Work out the finished part from the listing and answer in its coordinate system (mm). Coordinates: 2 decimals unless noted, no trailing zeros. Order: outer loops, then holes, each group sorted by start corner. A loop starts at its lowest first (then second) coordinate and runs counter-clockwise, first axis right, second up. Notation, with made-up numbers: M 79.5,9 L 102.5,9 A18 ccw 102.5,28 Z; hole C 41,-11 d3. An arc over 180 degrees is marked long. Use a Markdown table: item, result.
from build123d import *

# Parameters (mm, degrees)
SKETCH001_R     = 26
PAD_DEPTH       = 20
SKETCH002_R     = 15
POCKET_DEPTH    = 20.001
SKETCH_R        = 4
POCKET001_DEPTH = 26


with BuildPart() as part:
    # Sketch001 → Pad (new body)
    with BuildSketch(Plane.XY):
        Circle(SKETCH001_R)
    extrude(amount=PAD_DEPTH)

    # Sketch002 (on Face3 of Pad) → Pocket (cut, through all)
    with BuildSketch(Plane.XY.offset(20)):
        Circle(SKETCH002_R)
    extrude(amount=-POCKET_DEPTH, mode=Mode.SUBTRACT)

    # Sketch (on DatumPlane) → Pocket001 (cut)
    with BuildSketch(Plane.XZ.offset(26)):
        with Locations((0, 10)):
            Circle(SKETCH_R)
    extrude(amount=-POCKET001_DEPTH, mode=Mode.SUBTRACT)


solid = part.part
(1) A cutting plane is placed at B-B (x = 0). Determine the outline of the cut face in (y, z), then the cut area to 3 significant figures.
Conclusion:
| item | result |
|---|---|
| outline | M -26,0 L -15,0 L -15,6 L -26,6 Z; M -26,14 L -15,14 L -15,20 L -26,20 Z; M 15,0 L 26,0 L 26,20 L 15,20 Z |
| area | 352 mm2 |
(2) Given P1, Ø2, axis at y = -7, z = 9.5, coming from the +X side; P2, Ø10, axis at x = -15, z = 10, coming from the -Y side; P3, Ø10, axis at x = -9, z = 8.5, coming from the -Y side, each flat-ended and moving along its own axis, determine where each tip first touches the part or whether it passes through.
Conclusion:
| item | result |
|---|---|
| P1 | x = 25.3 |
| P2 | y = -24 |
| P3 | y = -25.69 |
(3) A cutting plane is placed at A-A (y = 0). Determine the outline of the cut face in (x, z).
Conclusion:
| item | result |
|---|---|
| outline | M -26,0 L -15,0 L -15,20 L -26,20 Z; M 15,0 L 26,0 L 26,20 L 15,20 Z |
(4) Straight lines are drawn through the part: L1, parallel to Y at x = -0.5, z = 1.75; L2, parallel to Z at x = 0, y = -18; L3, parallel to X at y = 12, z = 13.5. For each, find the intervals that lie inside material, in ascending order.
Conclusion:
| item | result |
|---|---|
| L1 | -26 to -14.99, 14.99 to 26 |
| L2 | 0 to 6, 14 to 20 |
| L3 | -23.07 to -9, 9 to 23.07 |
(5) A cutting plane is placed at C-C (x = -10.5). Determine the outline of the cut face in (y, z), then the cut area to 3 significant figures.
Conclusion:
| item | result |
|---|---|
| outline | M -23.79,0 L -10.71,0 L -10.71,20 L -23.79,20 Z; M 10.71,0 L 23.79,0 L 23.79,20 L 10.71,20 Z |
| area | 523 mm2 |
(6) A cutting plane is placed at D-D (z = 10). Determine the outline of the cut face in (x, y).
Conclusion:
| item | result |
|---|---|
| outline | M -4,-25.69 L -4,-14.46 A15 cw long 4,-14.46 L 4,-25.69 A26 ccw long Z |
(7) Determine the mould class of faces 1 (the cylindrical face through (2.15, -20.31, 13.373)), 2 (the flat face through (11, -11, 0)), 3 (the flat face through (11, -11, 20)) for opening direction Z: pulls with the +Z half, pulls with the -Z half, needs draft (parallel to the pull), parting line crosses it, or undercut.
Conclusion:
| item | result |
|---|---|
| face 1 | undercut |
| face 2 | pulls with the -Z half |
| face 3 | pulls with the +Z half |
